```python
from build123d import *

# Parameters (mm, degrees)
MODEL_R             = 3.6
MODEL_R_2           = 2.725
MODEL_R_3           = 2.5
BOSS_EXTRUDE1_DEPTH = 3


with BuildPart() as part:
    # Model → Boss-Extrude1 (new body)
    with BuildSketch(Plane.XY):
        with BuildLine():
            Line((-66.64035, 0), (66.64035, 0))
            ThreePointArc((66.64035, 0), (69.016228785, 0.984121215), (70.00035, 3.36))
            Line((70.00035, 3.36), (70.00035, 21.1105))
            Line((70.00035, 21.1105), (69.86629813, 22.498114684))
            Line((69.86629813, 22.498114684), (69.446311232, 23.988387428))
            Line((69.446311232, 23.988387428), (68.733529412, 25.548929055))
            Line((68.733529412, 25.548929055), (67.734761359, 27.16155254))
            Line((67.734761359, 27.16155254), (58.431673409, 40.525169242))
            ThreePointArc((58.431673409, 40.525169242), (58.118153534, 41.164216889), (58.01035, 41.867818343))
            Line((58.01035, 41.867818343), (58.01035, 65.939651469))
            ThreePointArc((58.01035, 65.939651469), (58.11831888, 66.643779624), (58.432304432, 67.283206562))
            Line((58.432304432, 67.283206562), (66.78383855, 79.267931576))
            Line((66.78383855, 79.267931576), (67.914068691, 81.051661321))
            Line((67.914068691, 81.051661321), (68.763177176, 82.764680123))
            Line((68.763177176, 82.764680123), (69.316681884, 84.394671222))
            Line((69.316681884, 84.394671222), (69.565395366, 85.915970428))
            Line((69.565395366, 85.915970428), (69.519060346, 87.308284697))
            Line((69.519060346, 87.308284697), (67.30949192, 103.030180971))
            Line((67.30949192, 103.030180971), (66.999561947, 104.350057085))
            Line((66.999561947, 104.350057085), (66.487504991, 105.437863083))
            Line((66.487504991, 105.437863083), (65.782163484, 106.319853558))
            Line((65.782163484, 106.319853558), (64.875433482, 107.017560512))
            Line((64.875433482, 107.017560512), (46.0351373, 118.337952538))
            ThreePointArc((46.0351373, 118.337952538), (45.285845094, 119.055243779), (44.918346815, 120.025238907))
            Line((44.918346815, 120.025238907), (40.094015429, 154.352140382))
            ThreePointArc((40.094015429, 154.352140382), (35.836168672, 162.70125074), (27.337884769, 166.652968529))
            ThreePointArc((27.337884769, 166.652968529), (26.108825382, 167.158066229), (25.350203438, 168.24903067))
            Line((25.350203438, 168.24903067), (24.828755998, 169.817409171))
            ThreePointArc((24.828755998, 169.817409171), (24.117671094, 170.371357056), (24.355513409, 171.2408))
            ThreePointArc((24.355513409, 171.2408), (22.368316822, 175.612570409), (17.911140334, 177.4))
            Line((17.911140334, 177.4), (7.437786988, 177.4))
            ThreePointArc((7.437786988, 177.4), (6.567071518, 177.232740152), (5.820301357, 176.754769847))
            Line((5.820301357, 176.754769847), (3.50035, 174.5536))
            ThreePointArc((3.50035, 174.5536), (3.500375, 173.207275), (4.8467, 173.2073))
            Line((4.8467, 173.2073), (7.50035, 173.2073))
            ThreePointArc((7.50035, 173.2073), (11.50035, 169.2073), (7.50035, 165.2073))
            Line((7.50035, 165.2073), (-7.49965, 165.2073))
            ThreePointArc((-7.49965, 165.2073), (-11.49965, 169.2073), (-7.49965, 173.2073))
            Line((-7.49965, 173.2073), (-4.846, 173.2073))
            ThreePointArc((-4.846, 173.2073), (-3.499675, 173.207275), (-3.49965, 174.5536))
            Line((-3.49965, 174.5536), (-5.819601357, 176.754769848))
            ThreePointArc((-5.819601357, 176.754769848), (-6.566371518, 177.232740152), (-7.437086988, 177.4))
            Line((-7.437086988, 177.4), (-17.910440334, 177.4))
            ThreePointArc((-17.910440334, 177.4), (-22.367616822, 175.612570409), (-24.354813409, 171.2408))
            ThreePointArc((-24.354813409, 171.2408), (-24.116971094, 170.371357056), (-24.828055998, 169.817409171))
            Line((-24.828055998, 169.817409171), (-25.349503438, 168.24903067))
            ThreePointArc((-25.349503438, 168.24903067), (-26.108125382, 167.158066229), (-27.337184769, 166.652968529))
            ThreePointArc((-27.337184769, 166.652968529), (-35.835468672, 162.70125074), (-40.093315429, 154.352140382))
            Line((-40.093315429, 154.352140382), (-44.917646815, 120.025238907))
            ThreePointArc((-44.917646815, 120.025238907), (-45.285145095, 119.055243779), (-46.0344373, 118.337952538))
            Line((-46.0344373, 118.337952538), (-64.874733482, 107.017560512))
            Line((-64.874733482, 107.017560512), (-65.764454542, 106.336263813))
            Line((-65.764454542, 106.336263813), (-66.464064741, 105.473352073))
            Line((-66.464064741, 105.473352073), (-66.989930499, 104.37360872))
            Line((-66.989930499, 104.37360872), (-67.307930284, 103.030180971))
            Line((-67.307930284, 103.030180971), (-69.517498709, 87.308284697))
            Line((-69.517498709, 87.308284697), (-69.564336548, 85.915534746))
            Line((-69.564336548, 85.915534746), (-69.316250952, 84.392453689))
            Line((-69.316250952, 84.392453689), (-68.763104771, 82.761395172))
            Line((-68.763104771, 82.761395172), (-67.914669475, 81.049208688))
            Line((-67.914669475, 81.049208688), (-66.785659136, 79.267931576))
            Line((-66.785659136, 79.267931576), (-58.427548106, 67.280305558))
            ThreePointArc((-58.427548106, 67.280305558), (-58.113308938, 66.640672262), (-58.00525, 65.936257417))
            Line((-58.00525, 65.936257417), (-58.00525, 41.865084223))
            ThreePointArc((-58.00525, 41.865084223), (-58.113143434, 41.161196344), (-58.426916507, 40.521942406))
            Line((-58.426916507, 40.521942406), (-67.732826699, 27.16155254))
            Line((-67.732826699, 27.16155254), (-68.732119035, 25.548966105))
            Line((-68.732119035, 25.548966105), (-69.445294681, 23.988426858))
            Line((-69.445294681, 23.988426858), (-69.86552208, 22.498130488))
            Line((-69.86552208, 22.498130488), (-69.99965, 21.1105))
            Line((-69.99965, 21.1105), (-69.99965, 3.3593))
            ThreePointArc((-69.99965, 3.3593), (-69.01573381, 0.98391619), (-66.64035, 0))
        make_face()
        with Locations((-56.49965, 13.52)):
            Circle(MODEL_R, mode=Mode.SUBTRACT)
        with Locations((-17.89965, 169.2073)):
            Circle(MODEL_R_2, mode=Mode.SUBTRACT)
        with Locations((-33.79965, 138.65)):
            Circle(MODEL_R_2, mode=Mode.SUBTRACT)
        with Locations((-56.49965, 93.22)):
            Circle(MODEL_R_3, mode=Mode.SUBTRACT)
        with Locations((56.50035, 13.52)):
            Circle(MODEL_R, mode=Mode.SUBTRACT)
        with Locations((17.90035, 169.2073)):
            Circle(MODEL_R_2, mode=Mode.SUBTRACT)
        with Locations((33.80035, 138.65)):
            Circle(MODEL_R_2, mode=Mode.SUBTRACT)
        with Locations((56.50035, 93.22)):
            Circle(MODEL_R_3, mode=Mode.SUBTRACT)
        with BuildLine():
            Line((-19.80285, 25.0481), (19.80355, 25.0481))
            ThreePointArc((19.80355, 25.0481), (31.150351096, 29.748098904), (35.85035, 41.0949))
            Line((35.85035, 41.0949), (35.85035, 66.7013))
            ThreePointArc((35.85035, 66.7013), (31.150351096, 78.048101096), (19.80355, 82.7481))
            Line((19.80355, 82.7481), (-19.80285, 82.7481))
            ThreePointArc((-19.80285, 82.7481), (-31.149651096, 78.048101096), (-35.84965, 66.7013))
            Line((-35.84965, 66.7013), (-35.84965, 41.0949))
            ThreePointArc((-35.84965, 41.0949), (-31.149651096, 29.748098904), (-19.80285, 25.0481))
        make_face(mode=Mode.SUBTRACT)
        with BuildLine():
            Line((-26.10965, 157.54), (-26.10965, 148.54))
            ThreePointArc((-26.10965, 148.54), (-23.56965, 146), (-21.02965, 148.54))
            Line((-21.02965, 148.54), (-21.02965, 157.54))
            ThreePointArc((-21.02965, 157.54), (-23.56965, 160.08), (-26.10965, 157.54))
        make_face(mode=Mode.SUBTRACT)
        with BuildLine():
            Line((-26.10965, 110.4), (-26.10965, 101.4))
            ThreePointArc((-26.10965, 101.4), (-23.56965, 98.86), (-21.02965, 101.4))
            Line((-21.02965, 101.4), (-21.02965, 110.4))
            ThreePointArc((-21.02965, 110.4), (-23.56965, 112.94), (-26.10965, 110.4))
        make_face(mode=Mode.SUBTRACT)
        with BuildLine():
            Line((-12.49965, 134.47), (-12.49965, 124.47))
            ThreePointArc((-12.49965, 124.47), (0.00035, 111.97), (12.50035, 124.47))
            Line((12.50035, 124.47), (12.50035, 134.47))
            ThreePointArc((12.50035, 134.47), (0.00035, 146.97), (-12.49965, 134.47))
        make_face(mode=Mode.SUBTRACT)
        with BuildLine():
            Line((21.03035, 157.54), (21.03035, 148.54))
            ThreePointArc((21.03035, 148.54), (23.57035, 146), (26.11035, 148.54))
            Line((26.11035, 148.54), (26.11035, 157.54))
            ThreePointArc((26.11035, 157.54), (23.57035, 160.08), (21.03035, 157.54))
        make_face(mode=Mode.SUBTRACT)
        with BuildLine():
            Line((21.03035, 110.4), (21.03035, 101.4))
            ThreePointArc((21.03035, 101.4), (23.57035, 98.86), (26.11035, 101.4))
            Line((26.11035, 101.4), (26.11035, 110.4))
            ThreePointArc((26.11035, 110.4), (23.57035, 112.94), (21.03035, 110.4))
        make_face(mode=Mode.SUBTRACT)
    extrude(amount=BOSS_EXTRUDE1_DEPTH)


solid = part.part
```
The model under review builds one solid part; all positions refer to its coordinate system, in mm. A direction names the side the tool comes from. Give positions to 0.01 mm unless a question says otherwise; leave off trailing zeros. Write each loop counter-clockwise with the first axis right and the second up, starting at its lowest first coordinate (ties: lowest second). Pieces come first, ordered by that corner, then holes. Notation, with made-up numbers: (14, 23) - (53, 23) arc R18 ccw to (53, 29) - close; hole circle Ø8 at (32.25, 36.25). An arc over 180 degrees is marked (long way). Answer in a Markdown table with one row per item. Add a question column.
1. We need section C-C on y = 93.22. Write out the cut boundary in (x, z).
2. Draft analysis for pull direction X (two halves, no side actions). For faces 3 (the flat face through (42.54, 136.95, 1.48)), 4 (the cylindrical face through (11.5, 169.3, 1.5)), 5 (the flat face through (-42.47, 137.43, 1.48)), 6 (the cylindrical face through (-31.3, 29.9, 1.5)), state which applies: +X half, -X half, draft (parallel to the pull), parting line (faces both ways), or undercut.
3. Insertion check: P1, Ø0.9, axis at y = 104.5, z = 2, coming from the +X side; P2, Ø1.5, axis at x = 0, z = 1, coming from the +Y side; P3, Ø0.9, axis at y = 153, z = 1, coming from the -X side. Each pin has a flat end and moves straight along its axis. Give the tip position at first contact, or say it passes through.
4. Wall thickness on line 1 along X through (y, z) = (57.5, 1.95); line 2 along X through (y, z) = (108.5, 0.9); line 3 along X through (y, z) = (15, 0.95): over which ranges is each line inside the solid? List them lowest first. Write a range as [from, to].
5. We need section B-B on y = 138.65. Write out the cut boundary in (x, z), then the cut area to 3 significant figures.
6. Tool access review of faces 1 (the cylindrical face through (0.275, 146.967, 1.479)), 2 (the flat face through (-1, 90, 0)): name each direction out of +Z, -Z, +X, -X, +Y, -Y from which nothing blocks a thin tool from reaching the whole face with its end or side.
7. We need section A-A on y = 63. Write out the cut boundary in (x, z).
8. We need section D-D on z = 1.6. State how many separate pieces and enclosed holes the cut face has, then the cut area to 3 significant figures.
Ans:
| question | item | result |
|---|---|---|
| 1 | outline | (-68.69, 0) - (-59, 0) - (-59, 3) - (-68.69, 3) - close; (-54, 0) - (54, 0) - (54, 3) - (-54, 3) - close; (59, 0) - (68.69, 0) - (68.69, 3) - (59, 3) - close |
| 2 | face 3 | +X half |
| 2 | face 4 | undercut |
| 2 | face 5 | -X half |
| 2 | face 6 | undercut |
| 3 | P1 | stops at x = 67.07 |
| 3 | P2 | stops at y = 165.21 |
| 3 | P3 | stops at x = -40.35 |
| 4 | line 1 | x = [-58.01, -35.85], [35.85, 58.01] |
| 4 | line 2 | x = [-62.41, -26.11], [-21.03, 21.03], [26.11, 62.41] |
| 4 | line 3 | x = [-70, -59.78], [-53.22, 53.22], [59.78, 70] |
| 5 | outline | (-42.3, 0) - (-36.52, 0) - (-36.52, 3) - (-42.3, 3) - close; (-31.07, 0) - (-11.78, 0) - (-11.78, 3) - (-31.07, 3) - close; (11.78, 0) - (31.08, 0) - (31.08, 3) - (11.78, 3) - close; (36.53, 0) - (42.3, 0) - (42.3, 3) - (36.53, 3) - close |
| 5 | area | 150 mm^2 |
| 6 | face 1 | +Z, -Z |
| 6 | face 2 | -Z, +X, -X, +Y, -Y |
| 7 | outline | (-58.01, 0) - (-35.85, 0) - (-35.85, 3) - (-58.01, 3) - close; (35.85, 0) - (58.01, 0) - (58.01, 3) - (35.85, 3) - close |
| 8 | separate pieces | 1 |
| 8 | enclosed holes | 14 |
| 8 | area | 14,300 mm^2 |
